Geometry: see drawing. Coordinates: mm, zero at the bounding-box minimum. Give positions to 0.01 mm unless a question says otherwise; leave off trailing zeros. Write each loop counter-clockwise with the first axis right and the second up, starting at its lowest first coordinate (ties: lowest second). Pieces come first, ordered by that corner, then holes. Notation, with made-up numbers: (-32, -17) -> (-15, -17) arc R27 cw to (-15, 9) -> close; hole circle Ø5 at (3, -38.75). An arc over 180 degrees is marked (long way). Answer as a JSON object with one key per item and string values. Group by question number.
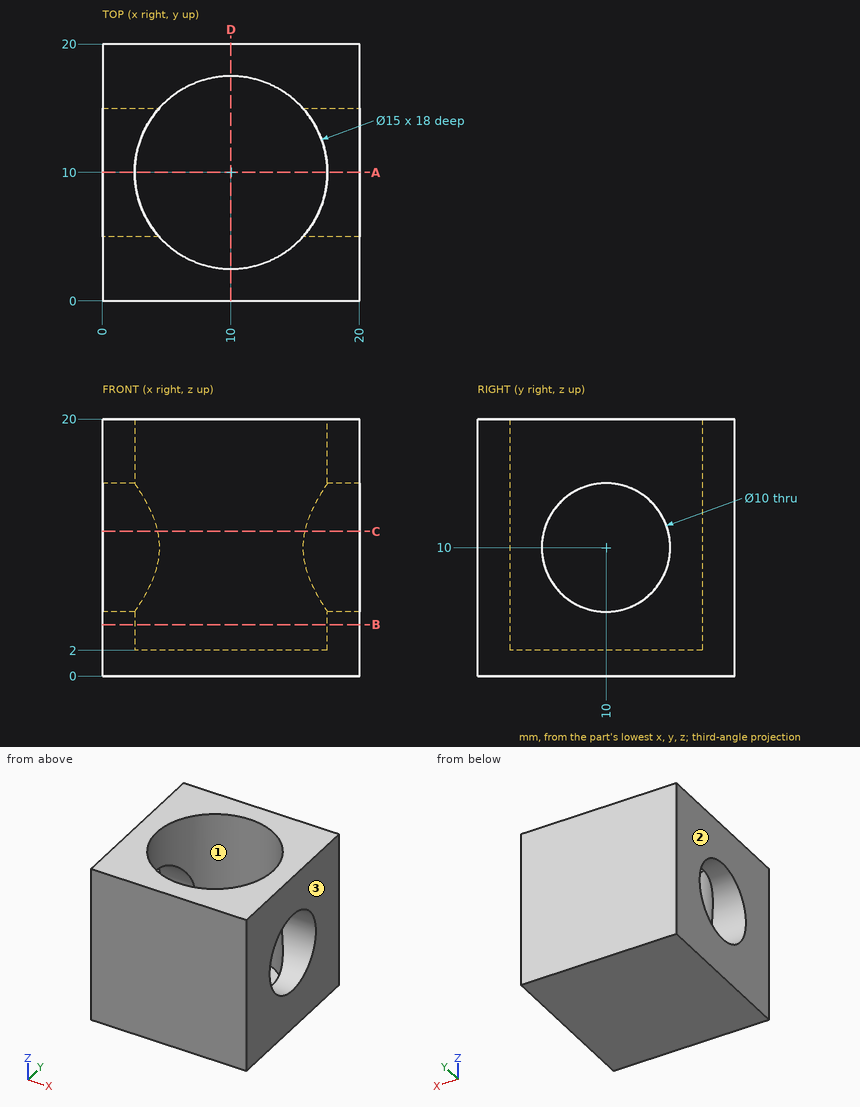
1. Section A-A (y = 10). Return the cut outline in (x, z), plus the area to 3 significant figures.
2. Mould query, pull axis X, two halves, no side actions, for the marked faces 1, 2 and 3. Classes: pulls with the +X half, pulls with the -X half, needs draft (parallel to the pull), parting line crosses it, or undercut.
3. Line query: line 1 (Y direction, x = 10, z = 8.5); line 2 (Y direction, x = 2.9, z = 10). Output: solid intervals per line, ascending.
4. Section D-D (x = 10). Return the cut outline in (y, z).
5. Section B-B (z = 4). Return the cut outline in (x, y).
6. Section C-C (z = 11.25). Return the cut outline in (x, y).
Working result:
{
 "1": {"outline": "(0, 0) -> (20, 0) -> (20, 5) -> (17.5, 5) -> (17.5, 2) -> (2.5, 2) -> (2.5, 5) -> (0, 5) -> close; (0, 15) -> (2.5, 15) -> (2.5, 20) -> (0, 20) -> close; (17.5, 15) -> (20, 15) -> (20, 20) -> (17.5, 20) -> close", "area": "80.0 mm^2"},
 "2": {"face 1": "undercut", "face 2": "pulls with the -X half", "face 3": "pulls with the +X half"},
 "3": {"line 1": "y = 0 to 2.5, 17.5 to 20", "line 2": "y = 0 to 5, 15 to 20"},
 "4": {"outline": "(0, 0) -> (20, 0) -> (20, 20) -> (17.5, 20) -> (17.5, 2) -> (2.5, 2) -> (2.5, 20) -> (0, 20) -> close"},
 "5": {"outline": "(0, 0) -> (20, 0) -> (20, 20) -> (0, 20) -> close; hole circle Ø15 at (10, 10)"},
 "6": {"outline": "(0, 0) -> (20, 0) -> (20, 5.16) -> (15.73, 5.16) arc R7.5 cw to (4.27, 5.16) -> (0, 5.16) -> close; (0, 14.84) -> (4.27, 14.84) arc R7.5 cw to (15.73, 14.84) -> (20, 14.84) -> (20, 20) -> (0, 20) -> close"}
}
